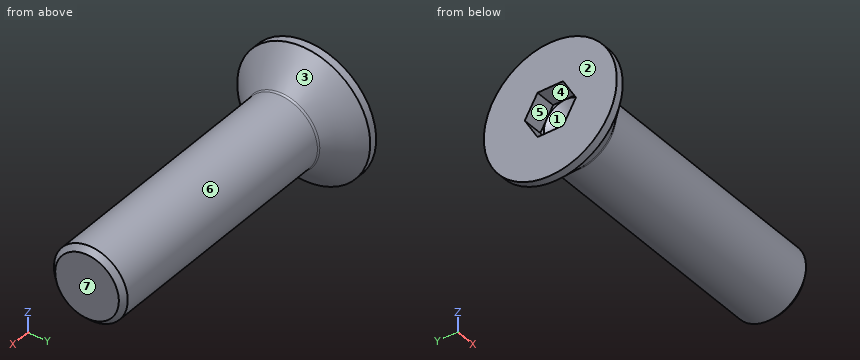
```python
from build123d import *

# Parameters (mm, degrees)
FILLET1_R   = 0.8
HEX_START   = -5.6
HEX_2_DEPTH = 5.6


with BuildPart() as part:
    # BodySke → BaseBody (revolve)
    with BuildSketch(Plane.XY, mode=Mode.PRIVATE) as basebody_sk:
        Polygon((0, 0), (0, 18.025), (2.135, 18.025), (10.16, 10), (78.626, 10), (80, 8.626), (80, 0), align=None)
    revolve(basebody_sk.sketch.rotate(Axis((0, 0, 0), (1, 0, 0)), 90), axis=Axis((0, 0, 0), (1, 0, 0)))

    # Fillet1
    fillet1_edges = [part.edges().sort_by_distance(p)[0] for p in [
        (10.16, 0, -10),
    ]]
    fillet(fillet1_edges, radius=FILLET1_R)

    # Hex 2: read off the stored shape, not the designer's step
    # Hex 2 outline → Hex 2 (cut)
    with BuildSketch(Plane.ZY.offset(HEX_START)):
        Polygon((-6, -3.464101615), (0, -6.92820323), (6, -3.464101615), (6, 3.464101615), (0, 6.92820323), (-6, 3.464101615), align=None)
    extrude(amount=HEX_2_DEPTH, mode=Mode.SUBTRACT)

    # Hex 2 2 outline → Hex 2 2 (revolve, cut)
    with BuildSketch(Plane.YX):
        Polygon((6, 5.6), (0, 9.064101615), (0, 5.6), align=None)
    revolve(axis=Axis((0, 0, 0), (1, 0, 0)), mode=Mode.SUBTRACT)


solid = part.part
```
Design review of the part built by this model. Coordinates are the model's own, in mm. Face numbers are marked on the shaded views. A direction names the side the tool comes from. Give positions to 0.01 mm unless a question says otherwise; leave off trailing zeros. Write each loop counter-clockwise with the first axis right and the second up, starting at its lowest first coordinate (ties: lowest second). Pieces come first, ordered by that corner, then holes. Notation, with made-up numbers: (6, -1) -> (15, -1) arc R19 cw to (15, 6) -> close; hole circle Ø11 at (77, -6). An arc over 180 degrees is marked (long way). Answer in a Markdown table with one row per item.
(1) To check wall thickness, follow probe 1 along Y at (x, z) = (47.5, -0.5); probe 2 along X at (y, z) = (3.5, -12). State the ranges of each line that lie inside material, in increasing order.
Results:
| item | result |
|---|---|
| probe 1 | -9.99 to 9.99 |
| probe 2 | 0 to 7.66 |
(2) Consider section A-A (x = 74). State the section outline as (y, z) points.
Results:
| item | result |
|---|---|
| outline | circle Ø20 at (0, 0) |
(3) For the marked faces 5, 6 and 7, list the 3-axis set-ups (+Z, -Z, +X, -X, +Y, -Y) from which the entire face can be reached by the end or side of a thin tool; tool diameter is ignored.
Results:
| item | result |
|---|---|
| face 5 | -X |
| face 6 | +X |
| face 7 | +Z, -Z, +X, +Y, -Y |
(4) Mouldability with a two-part tool opening along Y and no side actions: class the marked faces 1, 2, 3 and 4 as +Y half, -Y half, draft (parallel to the pull), parting line (faces both ways), or undercut.
Results:
| item | result |
|---|---|
| face 1 | undercut |
| face 2 | draft |
| face 3 | parting line |
| face 4 | undercut |
(5) Clearance check with flat-ended pins moving along their axes: pin 1 (10 mm diameter, centred on x = 32.5, z = 9, fed in from +Y); pin 2 (6 mm diameter, centred on x = 38.5, y = -9.5, fed in from +Z); pin 3 (1 mm diameter, centred on y = -3, z = -4, fed in from -X). State where each tip first meets the part, or that it passes through.
Results:
| item | result |
|---|---|
| pin 1 | y = 9.17 |
| pin 2 | z = 7.6 |
| pin 3 | x = 5.89 |
